Autodesk Inventor part; units mm, degrees
ref_plane "YZ Plane" through (0, 0, 0) normal (1, 0, 0) x (0, 1, 0)
ref_plane "XZ Plane" through (0, 0, 0) normal (0, 1, 0) x (-1, 0, 0)
ref_plane "XY Plane" through (0, 0, 0) normal (0, 0, 1) x (1, 0, 0)
sketch "Sketch1" plane through (0, 0, 0) normal (0, 0, 1) x (1, 0, 0)
  line L0 (0, 0) -> (0, 10)
  line L1 (0, 0) -> (4, 0)
  line L2 (4, 0) -> (4, 20) construction
  line L3 (4, 0) -> (0.3603, 10)
  line L4 (0, 10) -> (0.3603, 10)
  line L5 (0, 0) -> (15.4124, 0)
  dimension "d0" = 10
  dimension "d1" = 20
  dimension "d2" = 4
  dimension "d3" = 11.4123
  dimension "d4" = 20
revolve "Revolution1" add sketch "Sketch1" angle 360 about axis through (0, 0, 0) along (1, 0, 0)
sketch "Sketch2" plane through (0, 0, 0) normal (-1, 0, 0) x (0, 0, 1)
  circle A0 centre (0, 0) radius 10.25
  dimension "d6" = 20.5
extrude "Extrusion1" add sketch "Sketch2" along normal blind 1
sketch "Sketch3" plane through (-1, 0, 0) normal (-1, 0, 0) x (0, 0, 1)
  circle A0 centre (0, 0) radius 7.25
  dimension "d9" = 14.5
extrude "Extrusion2" add sketch "Sketch3" along normal blind 4
sketch "Sketch4" plane through (-5, 0, 0) normal (-1, 0, 0) x (0, 0, 1)
  circle A0 centre (0, 0) radius 13.75
  dimension "d12" = 27.5
extrude "Extrusion3" add sketch "Sketch4" along normal blind 80
sketch "Sketch5" plane through (-85, 0, 0) normal (-1, 0, 0) x (0, 0, 1)
  point P0 (0, 0)
  point P1 (0, 0)
hole "Hole1" at (-85, 0, 0) direction (1, 0, 0) diameter 8 depth 70 tip angle 118
properties part number "Jeringa_coreV2"
Part model, mm, in its own coordinate system. A direction names the side the tool comes from. Round coordinates to 2 decimals unless told otherwise and drop trailing zeros. Order: outer loops, then holes, each group sorted by start corner. A loop starts at its lowest first (then second) coordinate and runs counter-clockwise, first axis right, second up. Notation, with made-up numbers: M 54.5,-2 L 61.5,-2 A13 ccw 61.5,15 Z; hole C -18.75,-11.5 d3. An arc over 180 degrees is marked long. Answer in a Markdown table with one row per item. Add a question column.
Q1. Cut at B-B on x = -10.5. Give the cut face in (y, z).
Q2. Cut at A-A on x = -55.5. Give the cut face in (y, z).
Q3. Wall check: L1, parallel to Y at x = -59, z = 0; L2, parallel to Z at x = -78, y = -0.25; L3, parallel to Y at x = -16, z = -0.75. Give the ranges that are in metal, low to high. Write a range as from..to.
Q4. Pin check, flat tips, straight feed: pin 1 (3 mm diameter, centred on x = -9, y = -3.5, fed in from +Z); pin 2 (8 mm diameter, centred on x = -21.5, y = -8.5, fed in from +Z); pin 3 (6 mm diameter, centred on x = -23.5, y = -5.5, fed in from -Z). Stop position of each tip, or through.
Q5. 3-axis set-ups, long thin cutter, end or side, ignore diameter. For faces 4 (the face through (0.18, -2.17, -9.76)), 5 (the face through (-85, -3, 3)), 6 (the face through (-49.51, 3.905, -0.867)), 7 (the face through (-2.97, 6.43, 3.35)): which of +Z, -Z, +X, -X, +Y, -Y reach the whole face in a straight line?
Q6. Mould opens along Z. For faces 1 (the face through (-13.014, -0.678, -0.151)), 2 (the face through (-0.493, 10.006, -2.222)), 3 (the face through (-5, -6, 6)) say: +Z half, -Z half, draft (parallel to the pull), parting line (faces both ways), or undercut.
Established:
| question | item | result |
|---|---|---|
| 1 | outline | C 0,0 d27.5 |
| 2 | outline | C 0,0 d27.5; hole C 0,0 d8 |
| 3 | L1 | y = -13.75..-4, 4..13.75 |
| 3 | L2 | z = -13.75..-3.99, 3.99..13.75 |
| 3 | L3 | y = -13.73..-3.93, 3.93..13.73 |
| 4 | pin 1 | stops at z = 13.6 |
| 4 | pin 2 | stops at z = 12.99 |
| 4 | pin 3 | stops at z = -13.52 |
| 5 | face 4 | +X |
| 5 | face 5 | +Z, -Z, -X, +Y, -Y |
| 5 | face 6 | -X |
| 5 | face 7 | none |
| 6 | face 1 | undercut |
| 6 | face 2 | parting line |
| 6 | face 3 | draft |
